Read the model definition and answer for the solid it produces. Units are mm, in the model's axes. Coordinates: 2 decimals unless noted, no trailing zeros. Order: outer loops, then holes, each group sorted by start corner. A loop starts at its lowest first (then second) coordinate and runs counter-clockwise, first axis right, second up.
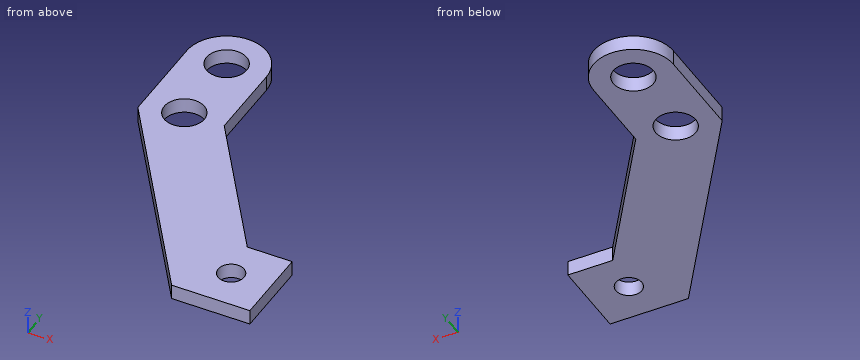
from build123d import *

# Parameters (mm, degrees)
SKETCH_1_R      = 2.6
SKETCH_1_R_2    = 4.025
EXTRUDE_1_DEPTH = 3


with BuildPart() as part:
    # ｽｹｯﾁ1 → ﾎﾞｽ - 押し出し1 (new body)
    with BuildSketch(Plane.XY):
        with BuildLine():
            Line((0, 46), (0, 27.508868037))
            Line((0, 27.508868037), (29.316460715, -15))
            Line((29.316460715, -15), (45, -15))
            Line((45, -15), (45, 1))
            Line((45, 1), (36, 1))
            Line((36, 1), (16, 30))
            Line((16, 30), (16, 46))
            ThreePointArc((16, 46), (8, 54), (0, 46))
        make_face()
        with Locations((37, -7)):
            Circle(SKETCH_1_R, mode=Mode.SUBTRACT)
        with Locations((8, 46)):
            Circle(SKETCH_1_R_2, mode=Mode.SUBTRACT)
        with Locations((8, 30)):
            Circle(SKETCH_1_R_2, mode=Mode.SUBTRACT)
    extrude(amount=EXTRUDE_1_DEPTH)


solid = part.part
Q1. The part is cut by section B-B, the plane y = -7. Determine the outline of the cut face in (x, z), then the cut area to 3 significant figures.
Q2. The part is cut by section A-A, the plane x = 37. Determine the outline of the cut face in (y, z).
Q3. The part is cut by section D-D, the plane x = 6.5. Determine the outline of the cut face in (y, z).
Q4. Straight lines are drawn through the part: L1, parallel to Y at x = 37, z = 1.1; L2, parallel to Y at x = 5.5, z = 1.9; L3, parallel to Y at x = 6.5, z = 1.15. For each, find the intervals that lie inside material, in ascending order.
Q5. The part is cut by section C-C, the plane z = 2. Determine the outline of the cut face in (x, y) (3 decimals).
Computed values:
1. outline: (23.8, 0) - (34.4, 0) - (34.4, 3) - (23.8, 3) - close; (39.6, 0) - (45, 0) - (45, 3) - (39.6, 3) - close
1. area: 48.0 mm2
2. outline: (-15, 0) - (-9.6, 0) - (-9.6, 3) - (-15, 3) - close; (-4.4, 0) - (1, 0) - (1, 3) - (-4.4, 3) - close
3. outline: (18.08, 0) - (26.26, 0) - (26.26, 3) - (18.08, 3) - close; (33.74, 0) - (42.26, 0) - (42.26, 3) - (33.74, 3) - close; (49.74, 0) - (53.86, 0) - (53.86, 3) - (49.74, 3) - close
4. L1: y = -15 to -9.6, -4.4 to 1
4. L2: y = 19.53 to 26.85, 33.15 to 42.85, 49.15 to 53.6
4. L3: y = 18.08 to 26.26, 33.74 to 42.26, 49.74 to 53.86
5. outline: (0, 27.509) - (29.316, -15) - (45, -15) - (45, 1) - (36, 1) - (16, 30) - (16, 46) arc R8 ccw to (0, 46) - close; hole circle Ø8.05 at (8, 30); hole circle Ø8.05 at (8, 46); hole circle Ø5.2 at (37, -7)
